Work out the finished part from the listing and answer in its coordinate system (mm). A direction names the side the tool comes from. Round coordinates to 2 decimals unless told otherwise and drop trailing zeros. Loops run counter-clockwise (first coordinate to the right, second up) from the corner with the lowest first, then second, coordinate; pieces in that order, holes last. Notation, with made-up numbers: (-8, 88) -> (48, 88) arc R32 cw to (48, 127) -> close; hole circle Ø1 at (-15.75, 82.25). An arc over 180 degrees is marked (long way). Write item = value, one per line. Start each with the question number.
```python
from build123d import *

# Parameters (mm, degrees)
F0_W     = 200
F0_H     = 200
F1_DEPTH = 70
F2_W     = 10
F2_H     = 200
F3_DEPTH = 100
F4_W     = 140
F4_H     = 45
F5_DEPTH = 50
F6_W     = 39
F6_H     = 140
F7_DEPTH = 90
F8_W     = 140
F8_H     = 60
F9_DEPTH = 59
F10_R    = 20
F11_R    = 40


with BuildPart() as f1:
    # F0 (on Right) → F1 (new body)
    with BuildSketch(Plane.YZ):
        Rectangle(F0_W, F0_H)
    extrude(amount=-F1_DEPTH)

    # F2 (on face) → F3 (cut)
    with BuildSketch(Plane(origin=(0, 0, -100), x_dir=(1, 0, 0), z_dir=(0, 0, -1))):
        with Locations((-5, 0)):
            Rectangle(F2_W, F2_H)
    extrude(amount=-F3_DEPTH, mode=Mode.SUBTRACT)

    # F4 (on face) → F5 (cut)
    with BuildSketch(Plane.YZ):
        with Locations((0, 22.5)):
            Rectangle(F4_W, F4_H)
    extrude(amount=-F5_DEPTH, mode=Mode.SUBTRACT)

    # F6 (on face) → F7 (cut)
    with BuildSketch(Plane.XY):
        with Locations((-30.5, 0)):
            Rectangle(F6_W, F6_H)
    extrude(amount=-F7_DEPTH, mode=Mode.SUBTRACT)

    # F8 (on face) → F9 (cut)
    with BuildSketch(Plane(origin=(-70, 0, 0), x_dir=(0, -1, 0), z_dir=(-1, 0, 0))):
        with Locations((0, -60)):
            Rectangle(F8_W, F8_H)
    extrude(amount=-F9_DEPTH, mode=Mode.SUBTRACT)

    # F10
    f10_edges = [f1.edges().sort_by_distance(p)[0] for p in [
        (-11, 0, -90),
    ]]
    fillet(f10_edges, radius=F10_R)

    # F11
    f11_edges = [f1.edges().sort_by_distance(p)[0] for p in [
        (-70, 0, 100),
    ]]
    fillet(f11_edges, radius=F11_R)


solid = f1.part
```
Item 1: Find the intervals of material crossed by line 1 along Y through (x, z) = (-24.5, 33); line 2 along X through (y, z) = (-29, -3.5); line 3 along X through (y, z) = (52.5, 44.5), in increasing order. Write a range as [from, to].
Item 2: Section C-C (x = -22) is taken. Determine the outline of the cut face in (y, z), then the cut area to 3 significant figures.
Item 3: The mould has two halves that part along Y. Classify faces 6 (the flat face through (-5, -85, 0)), 7 (the flat face through (-35, -100, -1)), 8 (the flat face through (-50, -1, 8)): pulls with the +Y half, pulls with the -Y half, needs draft (parallel to the pull), parting line crosses it, or undercut.
Item 4: Section B-B (z = -19) is taken. Determine the outline of the cut face in (x, y).
Item 5: Flat-ended cylindrical pins translate along their axes: pin 1 (8 mm diameter, centred on x = -4, y = 87.5, fed in from -Z); pin 2 (11.5 mm diameter, centred on x = -57, y = 10.5, fed in from +Z); pin 3 (10 mm diameter, centred on x = -59, y = -41, fed in from +Z). Find the tip coordinate at first contact, or state that the pin passes through.
Item 6: Section D-D (z = -40) is taken. Determine the outline of the cut face in (x, y).
Item 7: Section A-A (y = 58) is taken. Determine the outline of the cut face in (x, z), then the cut area to 3 significant figures.
Item 8: A tool of negligible diameter and unlimited length cuts with its end or side. For faces 1 (the flat face through (-5, 85, 0)), 2 (the flat face through (-35, -70, -23)), 3 (the flat face through (-25, -1, 45)), 4 (the cylindrical face through (-17.014, 0.98, -84.297)), 5 (the flat face through (-15, -1, 100)), from which of +Z, -Z, +X, -X, +Y, -Y can it reach the whole face along a straight path? Write none if from no direction.
Worked answers:
q1.line_1 = [-100, -70], [70, 100]
q1.line_2 = [-70, -50], [-11, -10]
q1.line_3 = [-70, -50]
q2.outline = (-100, -100) -> (100, -100) -> (100, 100) -> (-100, 100) -> close; hole (-70, -87.86) -> (70, -87.86) -> (70, 45) -> (-70, 45) -> close
q2.area = 21,400 mm2
q3.face_6 = needs draft
q3.face_7 = pulls with the -Y half
q3.face_8 = undercut
q4.outline = (-70, -100) -> (-10, -100) -> (-10, 100) -> (-70, 100) -> close; hole (-50, -70) -> (-11, -70) -> (-11, 70) -> (-50, 70) -> close
q5.pin_1 = 0
q5.pin_2 = 93.89
q5.pin_3 = 92
q6.outline = (-70, -100) -> (-10, -100) -> (-10, 100) -> (-70, 100) -> (-70, 70) -> (-11, 70) -> (-11, -70) -> (-70, -70) -> close
q7.outline = (-70, -100) -> (-10, -100) -> (-10, 0) -> (-11, 0) -> (-11, -70) arc R20 cw to (-31, -90) -> (-70, -90) -> close; (-70, -30) -> (-50, -30) -> (-50, 45) -> (0, 45) -> (0, 100) -> (-30, 100) arc R40 ccw to (-70, 60) -> close
q7.area = 5,780 mm2
q8.face_1 = -Z, +X, +Y, -Y
q8.face_2 = none
q8.face_3 = +X
q8.face_4 = -X
q8.face_5 = +Z, +X, -X, +Y, -Y
